Verification items for the finished model (mm, model axes). A direction names the side the tool comes from. Give positions to 0.01 mm unless a question says otherwise; leave off trailing zeros. Write each loop counter-clockwise with the first axis right and the second up, starting at its lowest first coordinate (ties: lowest second). Pieces come first, ordered by that corner, then holes. Notation, with made-up numbers: (-6, -37) -> (1, -37) arc R15 cw to (1, -32) -> close; hole circle Ø7 at (82, 25). An arc over 180 degrees is marked (long way). Answer as CSV lines item,"result". Start each with the question number.
1) Material ranges on L1, parallel to Z at x = 92.5, y = 1.75; L2, parallel to Z at x = 34, y = 4.25; L3, parallel to Z at x = 18.5, y = 4.5, recorded low to high.
2) Gauge pin test, flat ends, axial feed: pin 1 Ø3 at (y, z) = (3, 74) entering from +X; pin 2 Ø2 at (y, z) = (4, 19.5) entering from +X. Record the tip position at first contact, or that the pin passes through.
3) Sectioned sample at C-C on z = 26. Record the cut outline in (x, y), and give its area (3 significant figures).
4) Tool access check on faces 1 (the cylindrical face through (90.067, 3.131, 132.94)), 2 (the flat face through (32, 3.175, 70)). Record the directions out of +Z, -Z, +X, -X, +Y, -Y that give a thin tool (end or side, any length) a straight path to the whole face; none if there is none.
5) Mould release check, pull along Z, two halves, no side actions. Record for faces 3 (the flat face through (68, 0, 107)), 4 (the cylindrical face through (-26.16, 3.13, 6.14)): released by +Z, released by -Z, zero draft, split by the parting line, or undercut.
6) Sectioned sample at A-A on y = 1. Record the cut outline in (x, z), and give its area (3 significant figures).
7) Sectioned sample at B-B on x = 82. Record the cut outline in (y, z).
```python
from build123d import *

# Parameters (mm, degrees)
SKETCH1_R           = 2.2479
BOSS_EXTRUDE1_DEPTH = 6.35
CUT_EXTRUDE1_DEPTH  = 3.175


with BuildPart() as part:
    # Sketch1 → Boss-Extrude1 (new body)
    with BuildSketch(Plane(origin=(0, 0, 0), x_dir=(1, 0, 0), z_dir=(0, 1, 0))):
        with BuildLine():
            ThreePointArc((-22.298722012, -8.227846676), (-32.761767568, -1.823918477), (-26.902468415, -12.601405759))
            Line((-26.902468415, -12.601405759), (86.172305043, -131.627483084))
            ThreePointArc((86.172305043, -131.627483084), (96.635350599, -138.031411283), (90.776051446, -127.253924001))
            Line((90.776051446, -127.253924001), (-22.298722012, -8.227846676))
        make_face()
        with Locations(Location((92.261791516, -133.42766488, 0), (0, 0, 270))):
            Circle(SKETCH1_R, mode=Mode.SUBTRACT)
        with Locations(Location((-28.388208484, -6.42766488, 0), (0, 0, 270))):
            Circle(SKETCH1_R, mode=Mode.SUBTRACT)
    extrude(amount=BOSS_EXTRUDE1_DEPTH)

    # Sketch2 → Cut-Extrude1 (cut)
    with BuildSketch(Plane.XZ):
        Polygon((31.927377379, 65.307951298), (27.564134606, 69.934672098), (31.854628611, 74.63797054), (36.322762187, 69.934672148), align=None)
    extrude(amount=-CUT_EXTRUDE1_DEPTH, mode=Mode.SUBTRACT)


solid = part.part
```
Ans:
1,L1,"z = 127.08 to 131.19, 135.66 to 139.77"
1,L2,"z = 67.49 to 76.71"
1,L3,"z = 51.17 to 60.39"
2,pin 1,"stops at x = 41.61"
2,pin 2,"stops at x = -10.64"
3,outline,"(-14.17, 0) -> (-5.42, 0) -> (-5.42, 6.35) -> (-14.17, 6.35) -> close"
3,area,"55.6 mm²"
4,face 1,"+Y, -Y"
4,face 2,"-Y"
5,face 3,"zero draft"
5,face 4,"undercut"
6,outline,"(-26.9, 12.6) arc R6.35 ccw (long way) to (-22.3, 8.23) -> (31.93, 65.31) -> (27.56, 69.93) -> close; (31.94, 74.54) -> (36.32, 69.93) -> (90.78, 127.25) arc R6.35 ccw (long way) to (86.17, 131.63) -> close; hole circle Ø4.5 at (-28.39, 6.43); hole circle Ø4.5 at (92.26, 133.43)"
6,area,"1,220 mm²"
7,outline,"(0, 118.02) -> (6.35, 118.02) -> (6.35, 127.24) -> (0, 127.24) -> close"
